```python
from build123d import *

# Parameters (mm, degrees)
SKETCH1_W                                       = 5
SKETCH1_H                                       = 22
BOSS_EXTRUDE1_DEPTH                             = 65
SKETCH2_W                                       = 17.5
SKETCH2_H                                       = 95
SKETCH2_H_2                                     = 7
SKETCH2_W_2                                     = 15
BOSS_EXTRUDE2_DEPTH                             = 6
CSK_FOR_M3_FLAT_HEAD_MACHINE_SCREW1_D           = 3.4
CSK_FOR_M3_FLAT_HEAD_MACHINE_SCREW1_CSINK_D     = 6.3
CSK_FOR_M3_FLAT_HEAD_MACHINE_SCREW1_CSINK_ANGLE = 90
M3_CLEARANCE_HOLE2_AT_2_COUNT                   = 2
M3_CLEARANCE_HOLE2_AT_2_PITCH                   = 20
M3_CLEARANCE_HOLE2_AT_3_COUNT                   = 2
M3_CLEARANCE_HOLE2_AT_3_PITCH                   = 24.586378342
M3_CLEARANCE_HOLE2_AT_4_COUNT                   = 2
M3_CLEARANCE_HOLE2_AT_4_PITCH                   = 14.3
M3_CLEARANCE_HOLE2_AT_5_COUNT                   = 2
M3_CLEARANCE_HOLE2_AT_5_PITCH                   = 28.6
M3_CLEARANCE_HOLE2_AT_6_COUNT                   = 2
M3_CLEARANCE_HOLE2_AT_6_PITCH                   = 34.89928366
M3_CLEARANCE_HOLE2_AT_7_COUNT                   = 2
M3_CLEARANCE_HOLE2_AT_7_PITCH                   = 47.332969482
M3_CLEARANCE_HOLE2_AT_8_COUNT                   = 2
M3_CLEARANCE_HOLE2_AT_8_PITCH                   = 42.9
M3_CLEARANCE_HOLE2_AT_9_COUNT                   = 2
M3_CLEARANCE_HOLE2_AT_9_PITCH                   = 57.2
M3_CLEARANCE_HOLE2_AT_10_COUNT                  = 2
M3_CLEARANCE_HOLE2_AT_10_PITCH                  = 60.595709419
SKETCH8_R                                       = 2.165
CUT_EXTRUDE1_DEPTH                              = 5
RIB5_REACH                                      = 111.29
SKETCH9_WALL_W                                  = 240.579504986
SKETCH9_WALL_H                                  = 5
FILLET1_R                                       = 15
FILLET2_R                                       = 3
FILLET6_R                                       = 1
CHAMFER1_SIZE                                   = 1
CHAMFER2_SIZE                                   = 0.5


with BuildPart() as part:
    # Sketch1 → Boss-Extrude1 (new body)
    with BuildSketch(Plane(origin=(0, 0, 0), x_dir=(0, 0, -1), z_dir=(1, 0, 0))):
        with Locations((-2.5, 11)):
            Rectangle(SKETCH1_W, SKETCH1_H)
    extrude(amount=BOSS_EXTRUDE1_DEPTH)

    # Sketch2 → Boss-Extrude2 (add)
    with BuildSketch(Plane(origin=(0, 0, 0), x_dir=(1, 0, 0), z_dir=(0, 1, 0))):
        with Locations((23.75, 54.5)):
            Rectangle(SKETCH2_W, SKETCH2_H)
        with Locations((41.25, 54.5)):
            Rectangle(SKETCH2_W, SKETCH2_H)
        with Locations((41.25, 3.5)):
            Rectangle(SKETCH2_W, SKETCH2_H_2)
        with Locations((23.75, 3.5)):
            Rectangle(SKETCH2_W, SKETCH2_H_2)
        with Locations((7.5, 3.5)):
            Rectangle(SKETCH2_W_2, SKETCH2_H_2)
        with Locations((57.5, 3.5)):
            Rectangle(SKETCH2_W_2, SKETCH2_H_2)
    extrude(amount=BOSS_EXTRUDE2_DEPTH)

    # CSK for M3 Flat Head Machine Screw1 (through all)
    with Locations(Plane(origin=(0, 0, 0), x_dir=(-1, 0, 0), z_dir=(0, 0, -1))):
        with Locations((-55, 14), (-10, 14)):
            CounterSinkHole(CSK_FOR_M3_FLAT_HEAD_MACHINE_SCREW1_D / 2, CSK_FOR_M3_FLAT_HEAD_MACHINE_SCREW1_CSINK_D / 2, counter_sink_angle=CSK_FOR_M3_FLAT_HEAD_MACHINE_SCREW1_CSINK_ANGLE)

    # Sketch7 → M3 Clearance Hole2 (revolve, cut)
    with BuildSketch(Plane(origin=(22.5, 6, -30.5), x_dir=(0, 0, 1), z_dir=(1, 0, 0))):
        Polygon((0, 0), (0, 6), (2.2, 6), (1.7, 5.5), (1.7, 0), align=None)
    m3_clearance_hole2 = revolve(axis=Axis((22.5, 12.35, -30.5), (0, -1, 0)), mode=Mode.SUBTRACT)

    # M3 Clearance Hole2 at 2: M3 Clearance Hole2 ×2
    with Locations(*[(i * M3_CLEARANCE_HOLE2_AT_2_PITCH, 0, 0) for i in range(1, M3_CLEARANCE_HOLE2_AT_2_COUNT)]):
        add(m3_clearance_hole2, mode=Mode.SUBTRACT)

    # M3 Clearance Hole2 at 3: M3 Clearance Hole2 ×2
    with Locations(*[Vector(0.8134585631685806, 0, -0.5816228726655346) * (i * M3_CLEARANCE_HOLE2_AT_3_PITCH) for i in range(1, M3_CLEARANCE_HOLE2_AT_3_COUNT)]):
        add(m3_clearance_hole2, mode=Mode.SUBTRACT)

    # M3 Clearance Hole2 at 4: M3 Clearance Hole2 ×2
    with Locations(*[(0, 0, -i * M3_CLEARANCE_HOLE2_AT_4_PITCH) for i in range(1, M3_CLEARANCE_HOLE2_AT_4_COUNT)]):
        add(m3_clearance_hole2, mode=Mode.SUBTRACT)

    # M3 Clearance Hole2 at 5: M3 Clearance Hole2 ×2
    with Locations(*[(0, 0, -i * M3_CLEARANCE_HOLE2_AT_5_PITCH) for i in range(1, M3_CLEARANCE_HOLE2_AT_5_COUNT)]):
        add(m3_clearance_hole2, mode=Mode.SUBTRACT)

    # M3 Clearance Hole2 at 6: M3 Clearance Hole2 ×2
    with Locations(*[Vector(0.5730776652808003, 0, -0.8195010613515441) * (i * M3_CLEARANCE_HOLE2_AT_6_PITCH) for i in range(1, M3_CLEARANCE_HOLE2_AT_6_COUNT)]):
        add(m3_clearance_hole2, mode=Mode.SUBTRACT)

    # M3 Clearance Hole2 at 7: M3 Clearance Hole2 ×2
    with Locations(*[Vector(0.4225384593192284, 0, -0.9063449952397448) * (i * M3_CLEARANCE_HOLE2_AT_7_PITCH) for i in range(1, M3_CLEARANCE_HOLE2_AT_7_COUNT)]):
        add(m3_clearance_hole2, mode=Mode.SUBTRACT)

    # M3 Clearance Hole2 at 8: M3 Clearance Hole2 ×2
    with Locations(*[(0, 0, -i * M3_CLEARANCE_HOLE2_AT_8_PITCH) for i in range(1, M3_CLEARANCE_HOLE2_AT_8_COUNT)]):
        add(m3_clearance_hole2, mode=Mode.SUBTRACT)

    # M3 Clearance Hole2 at 9: M3 Clearance Hole2 ×2
    with Locations(*[(0, 0, -i * M3_CLEARANCE_HOLE2_AT_9_PITCH) for i in range(1, M3_CLEARANCE_HOLE2_AT_9_COUNT)]):
        add(m3_clearance_hole2, mode=Mode.SUBTRACT)

    # M3 Clearance Hole2 at 10: M3 Clearance Hole2 ×2
    with Locations(*[Vector(0.3300563718411858, 0, -0.943961223465791) * (i * M3_CLEARANCE_HOLE2_AT_10_PITCH) for i in range(1, M3_CLEARANCE_HOLE2_AT_10_COUNT)]):
        add(m3_clearance_hole2, mode=Mode.SUBTRACT)

    # Sketch8 → Cut-Extrude1 (cut)
    with BuildSketch(Plane(origin=(0, 6, 0), x_dir=(1, 0, 0), z_dir=(0, 1, 0))):
        with Locations(Location((22.5, 87.7, 0), (0, 0, 270))):
            Circle(SKETCH8_R)
        with Locations(Location((42.5, 87.7, 0), (0, 0, 270))):
            Circle(SKETCH8_R)
        with Locations(Location((22.5, 73.4, 0), (0, 0, 270))):
            Circle(SKETCH8_R)
        with Locations(Location((42.5, 73.4, 0), (0, 0, 270))):
            Circle(SKETCH8_R)
        with Locations(Location((22.5, 59.1, 0), (0, 0, 270))):
            Circle(SKETCH8_R)
        with Locations(Location((42.5, 59.1, 0), (0, 0, 270))):
            Circle(SKETCH8_R)
        with Locations(Location((22.5, 44.8, 0), (0, 0, 270))):
            Circle(SKETCH8_R)
        with Locations(Location((42.5, 44.8, 0), (0, 0, 270))):
            Circle(SKETCH8_R)
        with Locations(Location((22.5, 30.5, 0), (0, 0, 270))):
            Circle(SKETCH8_R)
        with Locations(Location((42.5, 30.5, 0), (0, 0, 270))):
            Circle(SKETCH8_R)
    extrude(amount=-CUT_EXTRUDE1_DEPTH, mode=Mode.SUBTRACT)

    # Sketch9 wall → Rib5 (add, up to next)
    with BuildSketch(Plane(origin=(32.5, 14, -6), x_dir=(0, -0.8, -0.6), z_dir=(0, 0.6, -0.8)), mode=Mode.PRIVATE) as rib5_sk1:
        Rectangle(SKETCH9_WALL_W, SKETCH9_WALL_H)
    rib5_tool1 = extrude(rib5_sk1.sketch, amount=-RIB5_REACH, mode=Mode.PRIVATE) - part.part
    add(rib5_tool1.solids().sort_by_distance((32.5, 14, -6))[0])

    # Fillet1
    fillet1_edges = [part.edges().sort_by_distance(p)[0] for p in [
        (50, 3, -7),
        (15, 3, -7),
    ]]
    fillet(fillet1_edges, radius=FILLET1_R - 0.0001)  # a hair under: the kernel refuses the full size

    # Fillet2
    fillet2_edges = [part.edges().sort_by_distance(p)[0] for p in [
        (65, 3, -7),
        (50, 3, -102),
        (15, 3, -102),
        (0, 3, -7),
        (0, 22, 2.5),
        (65, 22, 2.5),
    ]]
    fillet(fillet2_edges, radius=FILLET2_R)

    # Fillet6
    fillet6_edges = [part.edges().sort_by_distance(p)[0] for p in [
        (50, 6, 0),
        (15, 6, 0),
        (30, 6, -6),
        (32.5, 6, -12),
        (35, 6, -6),
    ]]
    fillet(fillet6_edges, radius=FILLET6_R)

    # Chamfer1
    chamfer1_edges = [part.edges().sort_by_distance(p)[0] for p in [
        (16.5, 22, 0),
        (50, 6, -60.49995),
        (15, 6, -60.49995),
        (11.45644013, 6, -12.317479289),
        (53.54355987, 6, -12.317479289),
        (32.5, 6, -102),
        (15.878679656, 6, -101.121320344),
        (49.121320344, 6, -101.121320344),
        (64.291283301, 6, -6.188242219),
        (0.708716699, 6, -6.188242219),
        (48.5, 22, 0),
        (64.121320344, 21.121320344, 0),
        (0.878679656, 21.121320344, 0),
        (0, 13, 0),
        (0, 6, -2.625872583),
        (65, 6, -2.625872583),
        (65, 13, 0),
        (0, 6.292893219, -0.292893219),
        (65, 6.292893219, -0.292893219),
    ]]
    chamfer(chamfer1_edges, length=CHAMFER1_SIZE)

    # Chamfer2
    chamfer2_edges = [part.edges().sort_by_distance(p)[0] for p in [
        (42.5, 6, -61.265),
        (22.5, 6, -46.965),
        (42.5, 6, -46.965),
        (22.5, 6, -32.665),
        (42.5, 6, -89.865),
        (22.5, 6, -75.565),
        (42.5, 6, -75.565),
        (22.5, 6, -61.265),
        (42.5, 6, -32.665),
        (22.5, 6, -89.865),
    ]]
    chamfer(chamfer2_edges, length=CHAMFER2_SIZE)


solid = part.part
```
Geometry: final body of the model. Coordinates: model frame, mm. A direction names the side the tool comes from. Coordinates: 2 decimals unless noted, no trailing zeros. Order: outer loops, then holes, each group sorted by start corner. A loop starts at its lowest first (then second) coordinate and runs counter-clockwise, first axis right, second up.
Item 1: Draft query along Z for faces 3 (the face through (50, 2, -60)), 4 (the face through (21.99, 0.75, -57.48)), 5 (the face through (64.4, 6.02, 0)). Return one class per face: released by +Z, released by -Z, zero draft, split by the parting line, or undercut.
Answer:
face 3: zero draft
face 4: undercut
face 5: released by -Z
Item 2: Contact query for flat-ended pins moving along their axis: P1, Ø5.5, axis at y = 2, z = -49.5, coming from the -X side; P2, Ø2, axis at x = 22, z = -88.5, coming from the +Y side; P3, Ø4.5, axis at x = 22.5, z = -73.4, coming from the +Y side (3 decimals). Output: stop coordinate, or through.
Answer:
P1: stops at x = 15
P2: stops at y = 1
P3: stops at y = 5.585
Item 3: Section query C-C (y = 9). Output: boundary loops of the cut face in (x, z), then the cut area to 3 significant figures.
Answer:
outline: (0, 1) - (1, 0) - (30, 0) - (30, -9.75) - (35, -9.75) - (35, 0) - (64, 0) - (65, 1) - (65, 5) - (0, 5) - close
area: 373 mm2
Item 4: Section query B-B (y = 14). Output: boundary loops of the cut face in (x, z).
Answer:
outline: (0, 1) - (1, 0) - (6.85, 0) - (8.3, 1.45) - (8.3, 5) - (0, 5) - close; (11.7, 1.45) - (13.15, 0) - (30, 0) - (30, -6) - (35, -6) - (35, 0) - (51.85, 0) - (53.3, 1.45) - (53.3, 5) - (11.7, 5) - close; (56.7, 1.45) - (58.15, 0) - (64, 0) - (65, 1) - (65, 5) - (56.7, 5) - close
Item 5: Section query A-A (z = -30.5). State how many separate pieces and enclosed holes the cut face has, then the cut area to 3 significant figures.
Answer:
separate pieces: 3
enclosed holes: 0
area: 158 mm2
Item 6: Material intervals for line 1 along X through (y, z) = (3.8, -30.5) (3 decimals); line 2 along Z through (x, y) = (42.5, 0.75); line 3 along X through (y, z) = (0.9, -30.5), sorted ascending.
Answer:
line 1: x = 15 to 20.335, 24.665 to 40.335, 44.665 to 50
line 2: z = -102 to -89.4, -86 to -75.1, -71.7 to -60.8, -57.4 to -46.5, -43.1 to -32.2, -28.8 to 5
line 3: x = 15 to 20.8, 24.2 to 40.8, 44.2 to 50
Item 7: Access query for faces 1 (the face through (41.67, 3.28, -71.4)), 2 (the face through (44, 0.8, -86.9)). Directions: +Z, -Z, +X, -X, +Y, -Y. A direction counts if a zero-diameter tool reaches every point of the face in a straight line with its end or side. Return the directions, or none.
Answer:
face 1: +Y
face 2: +Y, -Y
